Check sheet for the modelled part. Datum: model origin and axes. Units: mm. A direction names the side the tool comes from. Coordinates: 2 decimals unless noted, no trailing zeros. Loops run counter-clockwise (first coordinate to the right, second up) from the corner with the lowest first, then second, coordinate; pieces in that order, holes last.
```python
from build123d import *

# Parameters (mm, degrees)
F0_W     = 127
F0_H     = 127
F1_DEPTH = 76.2
F2_R     = 12.7
F3_T     = -6.35
F5_D     = 6.35


with BuildPart() as f1:
    # F0 (on Top) → F1 (new body)
    with BuildSketch(Plane.XY):
        with Locations((63.5, 63.5)):
            Rectangle(F0_W, F0_H)
    extrude(amount=F1_DEPTH)

    # F2
    f2_edges = [f1.edges().sort_by_distance(p)[0] for p in [
        (63.5, 0, 76.2),
    ]]
    fillet(f2_edges, radius=F2_R)

    # F3
    f3_openings = [f1.faces().sort_by_distance(p)[0] for p in [
        (127, 63.717753, 37.973421),
    ]]
    offset(amount=F3_T, openings=f3_openings)

    # F5 (through all)
    with Locations(Plane.XY.offset(76.2)):
        with Locations((52.258465, 54.398425), (68.767309, 76.650865), (88.000998, 53.506445)):
            Hole(F5_D / 2)


solid = f1.part
```
1) Section check B-B on z = 25. Enter the section's corners in (x, y), plus the area to 3 significant figures.
Answer sheet:
outline: (0, 0) - (127, 0) - (127, 6.35) - (6.35, 6.35) - (6.35, 120.65) - (127, 120.65) - (127, 127) - (0, 127) - close
area: 2,340 mm2
2) Depth check by flat-ended pin: pin 1 (8.5 mm diameter, centred on x = 88, y = 53.51, fed in from -Z); pin 2 (5 mm diameter, centred on x = 52.26, y = 54.4, fed in from -Z); pin 3 (19 mm diameter, centred on y = 67, z = 49.5, fed in from +X). Enter the tip coordinate at first touch or a pass-through.
Answer sheet:
pin 1: stops at z = 0
pin 2: passes through
pin 3: stops at x = 6.35
3) Section check A-A on x = 42. Enter the section's corners in (y, z), plus the area to 3 significant figures.
Answer sheet:
outline: (0, 0) - (127, 0) - (127, 76.2) - (12.7, 76.2) arc R12.7 ccw to (0, 63.5) - close; hole (6.35, 6.35) - (120.65, 6.35) - (120.65, 69.85) - (12.7, 69.85) arc R6.35 ccw to (6.35, 63.5) - close
area: 2,390 mm2
4) Section check C-C on y = 116.5. Enter the section's corners in (x, z).
Answer sheet:
outline: (0, 0) - (127, 0) - (127, 6.35) - (6.35, 6.35) - (6.35, 69.85) - (127, 69.85) - (127, 76.2) - (0, 76.2) - close
5) Set-up check for faces 5 (the flat face through (66, 67, 69.85)), 6 (the flat face through (63, 127, 38)): record each of +Z, -Z, +X, -X, +Y, -Y from which the full face is reachable in a straight line by a thin tool's end or side.
Answer sheet:
face 5: +X
face 6: +Z, -Z, +X, -X, +Y
6) Scan lines: line 1 (Z direction, x = 99, y = 82.5); line 2 (Y direction, x = 104, z = 32). Record each from-to range of solid material in increasing order.
Answer sheet:
line 1: z = 0 to 6.35, 69.85 to 76.2
line 2: y = 0 to 6.35, 120.65 to 127
7) Mould release check, pull along Z, two halves, no side actions. Record for faces 1 (the cylindrical face through (64.39, 3.62, 72.38)), 2 (the cylindrical face through (69.456, 73.551, 72.981)), 3 (the flat face through (6.35, 63, 38)), 4 (the cylindrical face through (67.52, 8.16, 67.94)): +Z half, -Z half, draft (parallel to the pull), parting line (faces both ways), or undercut.
Answer sheet:
face 1: +Z half
face 2: draft
face 3: undercut
face 4: undercut
